Can you work these out from the drawing? Everything is in mm from the part's minimum corner. A direction names the side the tool comes from. Give positions to 0.01 mm unless a question says otherwise; leave off trailing zeros. Write each loop counter-clockwise with the first axis right and the second up, starting at its lowest first coordinate (ties: lowest second). Pieces come first, ordered by that corner, then holes. Notation, with made-up numbers: (2.25, -16) - (41.25, -16) arc R24 ccw to (41.25, 3) - close; hole circle Ø1 at (-38.5, 23.25). An arc over 180 degrees is marked (long way). Write each question's results on one line, items separated by ' | '. Start each with the question number.
Item 1: Suppose I cut it at D-D on x = 19. List the corners of the cut face in (y, z) for me.
Item 2: We'd pull the mould along Y, two halves only. Please class the marked faces 1, 2 and 3: +Y half, -Y half, draft (parallel to the pull), parting line (faces both ways), or undercut.
Item 3: Suppose I cut it at C-C on z = 50.8. List the corners of the cut face in (x, y) for me.
Item 4: Please list where these lines run through material, in increasing order: line 1 along Z through (x, y) = (12.7, 0.8); line 2 along Y through (x, z) = (1.05, 12.7); line 3 along X through (y, z) = (8, 34).
Item 5: Will this pin go through, and if not, where does the flat tip stop? P1, Ø3, axis at x = 12.7, z = 50.8, coming from the -Y side.
Item 6: Suppose I cut it at A-A on x = 12.7. Count the separate pieces of the cut face and the enclosed holes in it, then the cut area to 3 significant figures.
Item 7: Suppose I cut it at B-B on y = 9. List the corners of the cut face in (x, z) for me.
Item 8: Which directions (+Z, -Z, +X, -X, +Y, -Y) give clear straight access to the entire face, cutting with the end or side of a thin tool? Please do the marked faces 4 and 5.
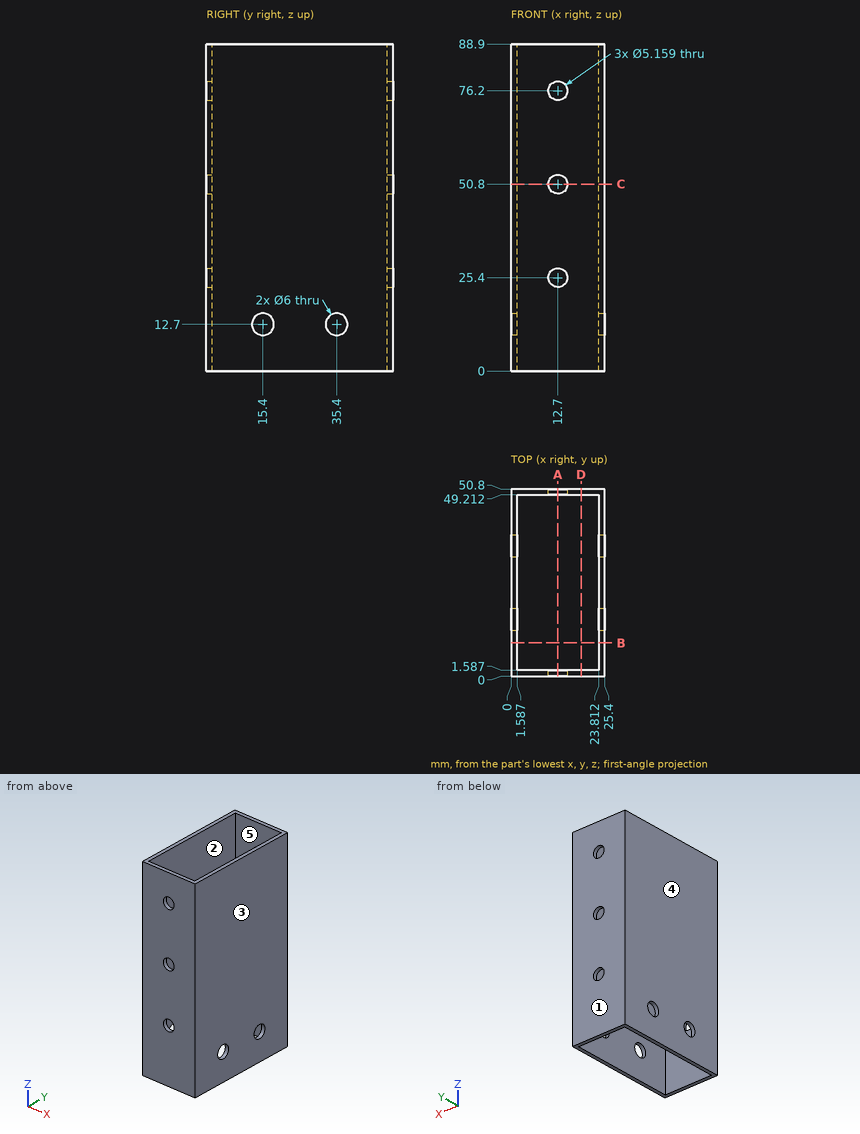
Checked values:
1) outline: (0, 0) - (1.59, 0) - (1.59, 88.9) - (0, 88.9) - close; (49.21, 0) - (50.8, 0) - (50.8, 88.9) - (49.21, 88.9) - close
2) face 1: +Y half | face 2: undercut | face 3: draft
3) outline: (0, 0) - (10.12, 0) - (10.12, 1.59) - (1.59, 1.59) - (1.59, 49.21) - (10.12, 49.21) - (10.12, 50.8) - (0, 50.8) - close; (15.28, 0) - (25.4, 0) - (25.4, 50.8) - (15.28, 50.8) - (15.28, 49.21) - (23.81, 49.21) - (23.81, 1.59) - (15.28, 1.59) - close
4) line 1: z = 0 to 22.82, 27.98 to 48.22, 53.38 to 73.62, 78.78 to 88.9 | line 2: y = 0 to 12.4, 18.4 to 32.4, 38.4 to 50.8 | line 3: x = 0 to 1.59, 23.81 to 25.4
5) P1: passes through
6) separate pieces: 8 | enclosed holes: 0 | area: 233 mm^2
7) outline: (0, 0) - (1.59, 0) - (1.59, 88.9) - (0, 88.9) - close; (23.81, 0) - (25.4, 0) - (25.4, 88.9) - (23.81, 88.9) - close
8) face 4: +Z, -Z, -X, +Y, -Y | face 5: +Z, -Z
